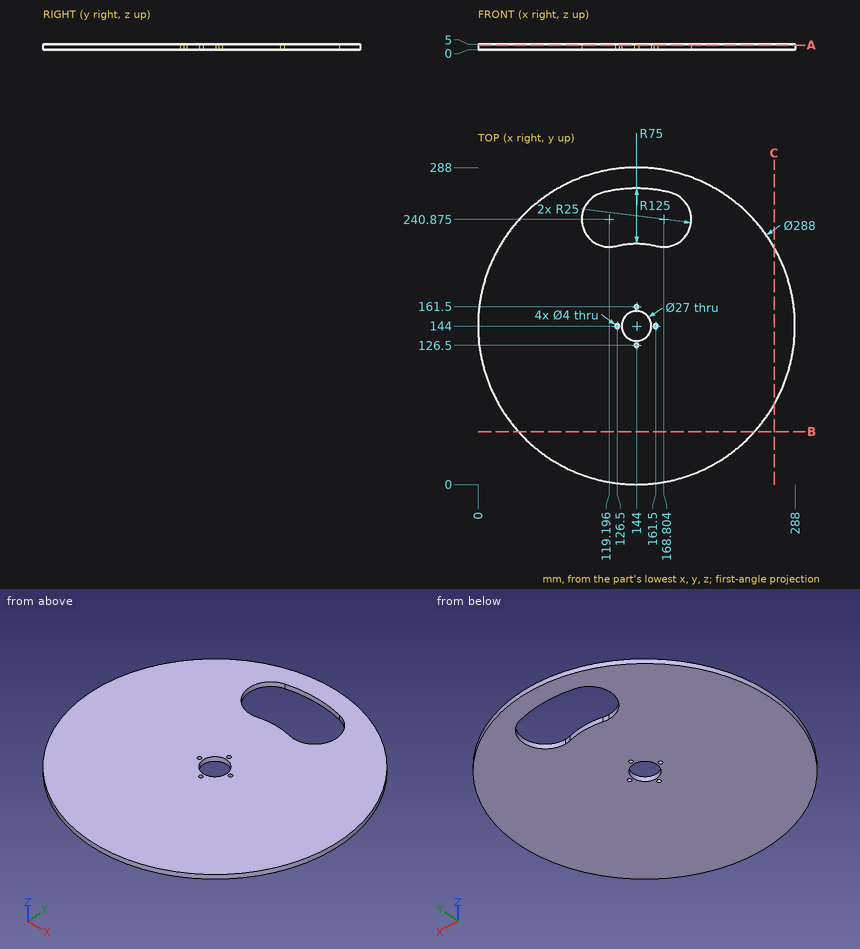
Answer from the drawing. Dimensions are ordinates in mm from the lowest x, y and z of the part. Give positions to 0.01 mm unless a question says otherwise; leave off trailing zeros. Loops run counter-clockwise (first coordinate to the right, second up) from the corner with the lowest first, then second, coordinate; pieces in that order, holes last. Notation, with made-up numbers: (-9, -37) - (49, -37) arc R18 ccw to (49, -25) - close; hole circle Ø9 at (77.5, 20.5). An arc over 180 degrees is marked (long way). Answer as CSV lines item,"result". Start each with the question number.
Item 1: A cutting plane is placed at A-A on z = 4.05. Determine the outline of the cut face in (x, y) (3 decimals).
Item 2: Find the intervals of material crossed by line 1 (X direction, y = 144, z = 1.2); line 2 (Y direction, x = 161.5, z = 3.75); line 3 (X direction, y = 161.5, z = 3.85), in increasing order. Write a range as from..to.
Item 3: Each of these flat-tipped pins is pushed along its axis until it touches: pin 1 (21.5 mm diameter, centred on x = 144, y = 144, fed in from -Z); pin 2 (3 mm diameter, centred on y = 204.5, z = 1, fed in from +X); pin 3 (3 mm diameter, centred on x = 183, z = 2, fed in from +Y); pin 4 (1.5 mm diameter, centred on y = 240, z = 3, fed in from +X). Where does it stop, or does it pass through?
Item 4: A cutting plane is placed at B-B on y = 48. Determine the outline of the cut face in (x, z), then the cut area to 3 significant figures.
Item 5: A cutting plane is placed at C-C on x = 269. Determine the outline of the cut face in (y, z).
Found:
1,outline,"circle Ø288 at (144, 144); hole (112.995, 265.094) arc R25 ccw to (125.397, 216.656) arc R75 cw to (162.603, 216.656) arc R25 ccw to (175.005, 265.094) arc R125 ccw to start; hole circle Ø4 at (126.5, 144); hole circle Ø27 at (144, 144); hole circle Ø4 at (144, 126.5); hole circle Ø4 at (144, 161.5); hole circle Ø4 at (161.5, 144)"
2,line 1,"x = 0..124.5, 128.5..130.5, 157.5..159.5, 163.5..288"
2,line 2,"y = 1.07..142, 146..216.93, 267.77..286.93"
2,line 3,"x = 1.07..142, 146..286.93"
3,pin 1,"passes through"
3,pin 2,"stops at x = 275.36"
3,pin 3,"stops at y = 283.03"
3,pin 4,"stops at x = 252"
4,outline,"(36.67, 0) - (251.33, 0) - (251.33, 5) - (36.67, 5) - close"
4,area,"1,070 mm^2"
5,outline,"(72.51, 0) - (215.49, 0) - (215.49, 5) - (72.51, 5) - close"
